```python
from build123d import *

# Parameters (mm, degrees)
SKETCH2_R = 0.65


with BuildPart() as part:
    # Sweep1: sweep along a path in Sketch1
    with BuildLine(Plane.XY) as sweep1_path:
        Line((-7, 5), (-4, 5))
        ThreePointArc((-4, 5), (-2.585786438, 4.414213562), (-2, 3))
        Line((-2, 3), (-2, 2))
        ThreePointArc((-2, 2), (-1.414213562, 0.585786438), (0, 0))
        Line((0, 0), (35.2, 0))
        ThreePointArc((35.2, 0), (36.614213562, 0.585786438), (37.2, 2))
        Line((37.2, 2), (37.2, 3))
        ThreePointArc((37.2, 3), (37.785786438, 4.414213562), (39.2, 5))
        Line((39.2, 5), (42.2, 5))
    # Sketch2 → Sweep1 (sweep)
    with BuildSketch(Plane(origin=(35.2, 0, 0), x_dir=(0, 0, -1), z_dir=(1, 0, 0))):
        Circle(SKETCH2_R)
    sweep(path=sweep1_path.line)


solid = part.part
```
The model under review builds one solid part; all positions refer to its coordinate system, in mm. A direction names the side the tool comes from. Round coordinates to 2 decimals unless told otherwise and drop trailing zeros. Loops run counter-clockwise (first coordinate to the right, second up) from the corner with the lowest first, then second, coordinate; pieces in that order, holes last. Notation, with made-up numbers: M 83,88 L 109,88 A31 cw 109,122 Z; hole C 31,-3.5 d11. An arc over 180 degrees is marked long. Answer as a JSON object with one key per item and string values.
(1) To check wall thickness, follow line 1 along X through (y, z) = (0.75, 0.35); line 2 along X through (y, z) = (1.5, 0.35); line 3 along Y through (x, z) = (22.5, 0). State the ranges of each line that lie inside material, in increasing order.
Resolved:
{"line 1": "-2.22 to -0.74, 35.94 to 37.42", "line 2": "-2.5 to -1.36, 36.56 to 37.7", "line 3": "-0.65 to 0.65"}
(2) Take a section at B-B on x = 11.5. Give the boundary of the cut face in (y, z).
Resolved:
{"outline": "C 0,0 d1.3"}
(3) Clearance check with flat-ended pins moving along their axes: P1, Ø1, axis at x = 30.5, y = 3, coming from the -Z side; P2, Ø3, axis at x = 20, y = 2, coming from the -Z side. State where each tip first meets the part, or that it passes through.
Resolved:
{"P1": "through", "P2": "z = -0.42"}
(4) Tool access review of faces 1 (the cylindrical face through (-5.479, 5.644, 0.085)), 2 (the flat face through (42.2, 5, 0)), 3 (the cylindrical face through (17.846, 0.644, 0.085)): name each direction out of +Z, -Z, +X, -X, +Y, -Y from which nothing blocks a thin tool from reaching the whole face with its end or side.
Resolved:
{"face 1": "-X", "face 2": "+Z, -Z, +X, +Y, -Y", "face 3": "none"}
(5) Draft analysis for pull direction X (two halves, no side actions). For faces 4 (the cylindrical face through (-2.635, 2.493, 0.141)), 5 (the flat face through (-7, 5, 0)), 6 (the cylindrical face through (40.721, 5.644, 0.085)), state which applies: released by +X, released by -X, zero draft, split by the parting line, or undercut.
Resolved:
{"face 4": "undercut", "face 5": "released by -X", "face 6": "zero draft"}
(6) Take a section at A-A on z = -0.15. Give the boundary of the cut face in (x, y).
Resolved:
{"outline": "M -7,4.37 L -4,4.37 A1.37 cw -2.63,3 L -2.63,2 A2.63 ccw 0,-0.63 L 35.2,-0.63 A2.63 ccw 37.83,2 L 37.83,3 A1.37 cw 39.2,4.37 L 42.2,4.37 L 42.2,5.63 L 39.2,5.63 A2.63 ccw 36.57,3 L 36.57,2 A1.37 cw 35.2,0.63 L 0,0.63 A1.37 cw -1.37,2 L -1.37,3 A2.63 ccw -4,5.63 L -7,5.63 Z"}
